from build123d import *

# Parameters (mm, degrees)
BOSS_EXTRUDE1_DEPTH = 3
SKETCH2_R           = 4.8
SKETCH2_R_2         = 3.375
CUT_EXTRUDE1_DEPTH  = 159.793104384
CUT_EXTRUDE3_DEPTH  = 159.793104384
CUT_EXTRUDE4_DEPTH  = 159.793104384
SKETCH8_R           = 3.5
CUT_EXTRUDE6_DEPTH  = 159.793104384
SKETCH12_R          = 1.5
CUT_EXTRUDE8_DEPTH  = 10
BOSS_EXTRUDE2_START = -3
BOSS_EXTRUDE2_DEPTH = 3


with BuildPart() as part:
    # Sketch1 → Boss-Extrude1 (new body)
    with BuildSketch(Plane(origin=(0, 0, 0), x_dir=(1, 0, 0), z_dir=(0, 1, 0))):
        with BuildLine():
            Line((140.3125, 17.497209599), (0.357142857, 19.99681097))
            ThreePointArc((0.357142857, 19.99681097), (-19.999202727, 0.178578547), (0, -20))
            Line((0, -20), (140, -17.5))
            ThreePointArc((140, -17.5), (157.499302386, -0.156256229), (140.3125, 17.497209599))
        make_face()
    extrude(amount=BOSS_EXTRUDE1_DEPTH)

    # Sketch2 → Cut-Extrude1 (cut, through all)
    with BuildSketch(Plane(origin=(0, 3, 0), x_dir=(1, 0, 0), z_dir=(0, 1, 0))):
        with Locations(Location((0, 0, 0), (0, 0, 270))):
            Circle(SKETCH2_R)
        with Locations(Location((140, 0, 0), (0, 0, 270))):
            Circle(SKETCH2_R_2)
    extrude(amount=-CUT_EXTRUDE1_DEPTH, mode=Mode.SUBTRACT)

    # Sketch4 → Cut-Extrude3 (cut, through all)
    with BuildSketch(Plane(origin=(0, 3, 0), x_dir=(1, 0, 0), z_dir=(0, 1, 0))):
        with BuildLine():
            ThreePointArc((101.494647455, -6.185682468), (107.64017994, 0.394224207), (101.283865867, 6.770744637))
            Line((101.283865867, 6.770744637), (29.173044697, 8.058643229))
            ThreePointArc((29.173044697, 8.058643229), (21.397292905, 0.29833633), (29.157599804, -7.477415462))
            Line((29.157599804, -7.477415462), (101.052392136, -6.193579885))
            Line((101.052392136, -6.193579885), (101.494647455, -6.185682468))
        make_face()
    extrude(amount=-CUT_EXTRUDE3_DEPTH, mode=Mode.SUBTRACT)

    # Sketch6 → Cut-Extrude4 (cut, through all)
    with BuildSketch(Plane(origin=(0, 0, 0), x_dir=(1, 0, 0), z_dir=(0, 1, 0))):
        with BuildLine():
            Line((-15.22, 0.75), (15.22, 0.75))
            ThreePointArc((15.22, 0.75), (15.97, 0), (15.22, -0.75))
            Line((15.22, -0.75), (-15.22, -0.75))
            ThreePointArc((-15.22, -0.75), (-15.97, 0), (-15.22, 0.75))
        make_face()
        with BuildLine():
            Line((-0.75, -9), (-0.75, 9))
            ThreePointArc((-0.75, 9), (0, 9.75), (0.75, 9))
            Line((0.75, 9), (0.75, -9))
            ThreePointArc((0.75, -9), (0, -9.75), (-0.75, -9))
        make_face()
    extrude(amount=CUT_EXTRUDE4_DEPTH, mode=Mode.SUBTRACT)

    # Sketch8 → Cut-Extrude6 (cut, through all)
    with BuildSketch(Plane(origin=(0, 3, 0), x_dir=(1, 0, 0), z_dir=(0, 1, 0))):
        Circle(SKETCH8_R)
        with Locations(Location((140, 0, 0), (0, 0, 270))):
            Circle(SKETCH8_R)
    extrude(amount=-CUT_EXTRUDE6_DEPTH, mode=Mode.SUBTRACT)

    # Sketch12 → Cut-Extrude8 (cut)
    with BuildSketch(Plane(origin=(0, 3, 0), x_dir=(1, 0, 0), z_dir=(0, 1, 0))):
        with Locations(Location((83.194560065, 10.922443863, 0), (0, 0, 270))):
            Circle(SKETCH12_R)
        with Locations(Location((34.541656008, 12.231474735, 0), (0, 0, 270))):
            Circle(SKETCH12_R)
        with Locations(Location((34.541656008, -12.373276524, 0), (0, 0, 270))):
            Circle(SKETCH12_R)
        with Locations(Location((81.871511394, -13.646710106, 0), (0, 0, 270))):
            Circle(SKETCH12_R)
    extrude(amount=-CUT_EXTRUDE8_DEPTH, mode=Mode.SUBTRACT)

    # Sketch14 → Boss-Extrude2 (add)
    with BuildSketch(Plane(origin=(0, 3, 0), x_dir=(1, 0, 0), z_dir=(0, 1, 0)).offset(BOSS_EXTRUDE2_START)):
        with BuildLine():
            Line((140.3125, 17.497209599), (142.86969749, 17.497209599))
            ThreePointArc((142.86969749, 17.497209599), (160.632042581, 0.214901924), (143.301107477, -17.5))
            Line((143.301107477, -17.5), (140, -17.5))
            ThreePointArc((140, -17.5), (157.499302386, -0.156256229), (140.3125, 17.497209599))
        make_face()
    extrude(amount=BOSS_EXTRUDE2_DEPTH)


solid = part.part
Design review of the part built by this model. Coordinates are the model's own, in mm. Round coordinates to 2 decimals unless told otherwise and drop trailing zeros. Order: outer loops, then holes, each group sorted by start corner. A loop starts at its lowest first (then second) coordinate and runs counter-clockwise, first axis right, second up.
1) Consider section C-C (x = 134.5). State the section outline as (y, z) points, plus the area to 3 significant figures.
The answers:
outline: (0, -17.6) - (3, -17.6) - (3, 17.6) - (0, 17.6) - close
area: 106 mm2
2) For L1, parallel to X at y = 1.15, z = -4; L2, parallel to X at y = 1.75, z = 0.5; L3, parallel to Z at x = 140, y = 0.9, list the stretches that pass through material, from the lowest coordinate up.
The answers:
L1: x = -19.6 to -2.65, 2.65 to 22.34, 106.47 to 160.17
L2: x = -19.99 to -15.78, 15.78 to 21.44, 107.59 to 136.54, 143.46 to 160.63
L3: z = -17.5 to -3.5, 3.5 to 17.5
3) Draft analysis for pull direction Z (two halves, no side actions). For faces 1 (the cylindrical face through (35, 1.5, 13.8)), 2 (the flat face through (72, 0, 9)), 3 (the cylindrical face through (-19.99, 1.48, -0.62)), 4 (the flat face through (-0.75, 1, -7)), state which applies: released by +Z, released by -Z, zero draft, split by the parting line, or undercut.
The answers:
face 1: undercut
face 2: zero draft
face 3: split by the parting line
face 4: undercut
4) Consider section A-A (y = 0.55). Count the separate pieces of the cut face and the enclosed holes in it, plus the area to 3 significant figures.
The answers:
separate pieces: 1
enclosed holes: 7
area: 5,100 mm2
5) Consider section B-B (x = 104.5). State the section outline as (y, z) points, plus the area to 3 significant figures.
The answers:
outline: (0, -18.14) - (3, -18.14) - (3, -5.84) - (0, -5.84) - close; (0, 5.27) - (3, 5.27) - (3, 18.13) - (0, 18.13) - close
area: 75.5 mm2
6) Clearance check with flat-ended pins moving along their axes: pin 1 Ø0.9 at (x, y) = (-8.5, 2) entering from -Z; pin 2 Ø1 at (y, z) = (0.5, -4) entering from -X; pin 3 Ø1.3 at (x, y) = (141, 1) entering from -Z. State where each tip first meets the part, or that it passes through.
The answers:
pin 1: stops at z = -18.31
pin 2: stops at x = -19.69
pin 3: stops at z = -17.5
